The model under review builds one solid part; all positions refer to its coordinate system, in mm. A direction names the side the tool comes from. Coordinates: 2 decimals unless noted, no trailing zeros. Write each loop counter-clockwise with the first axis right and the second up, starting at its lowest first coordinate (ties: lowest second). Pieces come first, ordered by that corner, then holes. Notation, with made-up numbers: (83.5, 89.25) -> (110.5, 89.25) arc R19 ccw to (110.5, 96.25) -> close; hole circle Ø8 at (2.5, -28). An arc over 180 degrees is marked (long way). Put each result on its own line as item: value. Start each with the question number.
from build123d import *

# Parameters (mm, degrees)
BOSS_EXTRUDE1_DEPTH   = 1.5
CHAMFER1_SIZE         = 1
F_1_0MM_DOWEL_HOLE1_D = 1


with BuildPart() as part:
    # Sketch1 → Boss-Extrude1 (new body)
    with BuildSketch(Plane.XY):
        with BuildLine():
            Line((0, 35.4625), (0, -35.4625))
            ThreePointArc((0, -35.4625), (1.464466094, -38.998033906), (5, -40.4625))
            Line((5, -40.4625), (7, -40.4625))
            ThreePointArc((7, -40.4625), (10.535533906, -38.998033906), (12, -35.4625))
            Line((12, -35.4625), (12, -32.9625))
            Line((12, -32.9625), (7.5, -32.9625))
            Line((7.5, -32.9625), (7.5, -31.305))
            Line((7.5, -31.305), (12, -31.305))
            Line((12, -31.305), (12, -26.805))
            Line((12, -26.805), (7.5, -26.805))
            Line((7.5, -26.805), (7.5, -25.2))
            Line((7.5, -25.2), (12, -25.2))
            Line((12, -25.2), (12, -20.7))
            Line((12, -20.7), (7.5, -20.7))
            Line((7.5, -20.7), (7.5, -19.1475))
            Line((7.5, -19.1475), (12, -19.1475))
            Line((12, -19.1475), (12, -14.6475))
            Line((12, -14.6475), (7.5, -14.6475))
            Line((7.5, -14.6475), (7.5, -13.1475))
            Line((7.5, -13.1475), (12, -13.1475))
            Line((12, -13.1475), (12, -8.6475))
            Line((12, -8.6475), (7.5, -8.6475))
            Line((7.5, -8.6475), (7.5, -7.2))
            Line((7.5, -7.2), (12, -7.2))
            Line((12, -7.2), (12, -2.7))
            Line((12, -2.7), (7.5, -2.7))
            Line((7.5, -2.7), (7.5, -1.305))
            Line((7.5, -1.305), (12, -1.305))
            Line((12, -1.305), (12, 3.195))
            Line((12, 3.195), (7.5, 3.195))
            Line((7.5, 3.195), (7.5, 4.5375))
            Line((7.5, 4.5375), (12, 4.5375))
            Line((12, 4.5375), (12, 9.0375))
            Line((12, 9.0375), (7.5, 9.0375))
            Line((7.5, 9.0375), (7.5, 10.3275))
            Line((7.5, 10.3275), (12, 10.3275))
            Line((12, 10.3275), (12, 14.8275))
            Line((12, 14.8275), (7.5, 14.8275))
            Line((7.5, 14.8275), (7.5, 16.065))
            Line((7.5, 16.065), (12, 16.065))
            Line((12, 16.065), (12, 20.565))
            Line((12, 20.565), (7.5, 20.565))
            Line((7.5, 20.565), (7.5, 21.75))
            Line((7.5, 21.75), (12, 21.75))
            Line((12, 21.75), (12, 26.25))
            Line((12, 26.25), (7.5, 26.25))
            Line((7.5, 26.25), (7.5, 27.3825))
            Line((7.5, 27.3825), (12, 27.3825))
            Line((12, 27.3825), (12, 31.8825))
            Line((12, 31.8825), (7.5, 31.8825))
            Line((7.5, 31.8825), (7.5, 32.9625))
            Line((7.5, 32.9625), (12, 32.9625))
            Line((12, 32.9625), (12, 35.4625))
            ThreePointArc((12, 35.4625), (10.535533906, 38.998033906), (7, 40.4625))
            Line((7, 40.4625), (5, 40.4625))
            ThreePointArc((5, 40.4625), (1.464466094, 38.998033906), (0, 35.4625))
        make_face()
    extrude(amount=BOSS_EXTRUDE1_DEPTH)

    # Chamfer1
    chamfer1_edges = [part.edges().sort_by_distance(p)[0] for p in [
        (12, 31.8825, 0.75),
        (12, 27.3825, 0.75),
        (12, 26.25, 0.75),
        (12, 21.75, 0.75),
        (12, 20.565, 0.75),
        (12, 16.065, 0.75),
        (12, 14.8275, 0.75),
        (12, 10.3275, 0.75),
        (12, 9.0375, 0.75),
        (12, 4.5375, 0.75),
        (12, 3.195, 0.75),
        (12, -1.305, 0.75),
        (12, -2.7, 0.75),
        (12, -7.2, 0.75),
        (12, -8.6475, 0.75),
        (12, -13.1475, 0.75),
        (12, -14.6475, 0.75),
        (12, -19.1475, 0.75),
        (12, -20.7, 0.75),
        (12, -25.2, 0.75),
        (12, -26.805, 0.75),
        (12, -31.305, 0.75),
        (12, -32.9625, 0.75),
        (12, 32.9625, 0.75),
    ]]
    chamfer(chamfer1_edges, length=CHAMFER1_SIZE)

    # Ø1.0mm Dowel Hole1 (through all)
    with Locations(Plane.XY.offset(1.5)):
        with Locations((7.712132034, 32.750367966), (7.712132034, 32.094632034), (7.712132034, 27.170367966), (7.712132034, 26.462132034), (7.712132034, 21.537867966), (7.712132034, 20.777132034), (7.712132034, 15.852867966), (7.712132034, 15.039632034), (7.712132034, 10.115367966), (7.712132034, 9.249632034), (7.712132034, 4.325367966), (7.712132034, 3.407132034), (7.712132034, -1.517132034), (7.712132034, -2.487867966), (7.712132034, -7.412132034), (7.712132034, -8.435367966), (7.712132034, -13.359632034), (7.712132034, -14.435367966), (7.712132034, -19.359632034), (7.712132034, -20.487867966), (7.712132034, -25.412132034), (7.712132034, -26.592867966), (7.712132034, -31.517132034), (7.712132034, -32.750367966)):
            Hole(F_1_0MM_DOWEL_HOLE1_D / 2)


solid = part.part
1. The part is to be moulded in two halves that separate along Y. For faces 1 (the flat face through (12, 1, 1)), 2 (the cylindrical face through (10.574, 38.959, 0.74)), 3 (the flat face through (10, 16.065, 1)), say which applies: released by +Y, released by -Y, zero draft, split by the parting line, or undercut.
2. Tool access review of faces 4 (the flat face through (10, -25.2, 1)), 5 (the flat face through (12, 30, 1)): name each direction out of +Z, -Z, +X, -X, +Y, -Y from which nothing blocks a thin tool from reaching the whole face with its end or side.
3. Consider section B-B on x = 2. State the section outline as (y, z) points, then the cut area to 3 significant figures.
4. Wall thickness on line 1 (X direction, y = -32, z = 1.25); line 2 (X direction, y = 33, z = 1); line 3 (X direction, y = 5.5, z = 1.1): over which ranges is each line inside the solid? List them lowest first. Write a range as from..to.
5. Consider section A-A on x = 9. State how many separate pieces and enclosed holes the cut face has, then the cut area to 3 significant figures.
6. Insertion check: P1, Ø0.8, axis at x = 9.5, z = 0.5, coming from the -Y side; P2, Ø0.8, axis at x = 10, z = 0.5, coming from the +Y side. Each pin has a flat end and moves straight along its axis. Give the tip position at first contact, or say it passes through.
Output values:
1. face 1: zero draft
1. face 2: released by +Y
1. face 3: undercut
2. face 4: +Z, -Z, +X
2. face 5: +Z, -Z, +X, +Y, -Y
3. outline: (-39.46, 0) -> (39.46, 0) -> (39.46, 1.5) -> (-39.46, 1.5) -> close
3. area: 118 mm^2
4. line 1: x = 0..7.5
4. line 2: x = 0..7.28, 8.15..11.04
4. line 3: x = 0..11.96
5. separate pieces: 13
5. enclosed holes: 0
5. area: 95.5 mm^2
6. P1: stops at y = -40
6. P2: stops at y = 39.73
